Can you work these out from the model? Positions are in its coordinate system, mm. Round coordinates to 2 decimals unless told otherwise and drop trailing zeros. Loops run counter-clockwise (first coordinate to the right, second up) from the corner with the lowest first, then second, coordinate; pieces in that order, holes last.
Autodesk Inventor part; units mm, degrees
ref_plane "YZ Plane" through (0, 0, 0) normal (1, 0, 0) x (0, 1, 0)
ref_plane "XZ Plane" through (0, 0, 0) normal (0, 1, 0) x (-1, 0, 0)
ref_plane "XY Plane" through (0, 0, 0) normal (0, 0, 1) x (1, 0, 0)
sketch "Sketch2" plane through (0, 0, 0) normal (0, 0, 1) x (1, 0, 0)
  line L0 (-7.3607, 82.5814) -> (-7.3607, 22.5627)
  line L1 (-7.3607, 22.5627) -> (0.6393, 28.1644)
  line L2 (0.6393, 28.1644) -> (0.6393, 82.5814)
  line L3 (-7.3607, 82.5814) -> (-10.3607, 82.5814)
  line L4 (-10.3607, 82.5814) -> (-10.3607, 100.5814)
  line L5 (0.6393, 82.5814) -> (3.6393, 82.5814)
  line L6 (3.6393, 82.5814) -> (3.6393, 100.5814)
  line L7 (-10.3607, 100.5814) -> (3.6393, 100.5814)
  line L8 (-10.3607, 85.5814) -> (3.6393, 85.5814) construction
  point P0 (0, 0)
  dimension "d3" = 125
  dimension "d9" = 8
  dimension "d10" = 18
  dimension "d11" = 3
  dimension "d12" = 57.417
  dimension "d13" = 3
  dimension "d14" = 18
extrude "Extrusion1" add sketch "Sketch2" along normal blind 3
sketch "Sketch3" plane through (0, 0, 3) normal (0, 0, 1) x (1, 0, 0)
  line L0 (-10.3607, 100.5814) -> (-10.3607, 82.5814)
  line L1 (3.6393, 82.5814) -> (3.6393, 100.5814)
  line L2 (-10.3607, 85.5814) -> (-7.3607, 85.5814)
  line L3 (-7.3607, 85.5814) -> (-7.3607, 97.5814)
  line L4 (-7.3607, 97.5814) -> (-10.3607, 97.5814)
  line L5 (-10.3607, 97.5814) -> (-10.3607, 85.5814)
  line L6 (3.6393, 85.5814) -> (0.6393, 85.5814)
  line L7 (0.6393, 85.5814) -> (0.6393, 97.5814)
  line L8 (0.6393, 97.5814) -> (3.6393, 97.5814)
  line L9 (3.6393, 97.5814) -> (3.6393, 85.5814)
  point P0 (0, 0)
  dimension "d15" = 3
  dimension "d16" = 12
  dimension "d17" = 3
extrude "Extrusion2" cut sketch "Sketch3" against normal through all
equation "\"d14\" = d10"
properties part number "k2_t_leg"
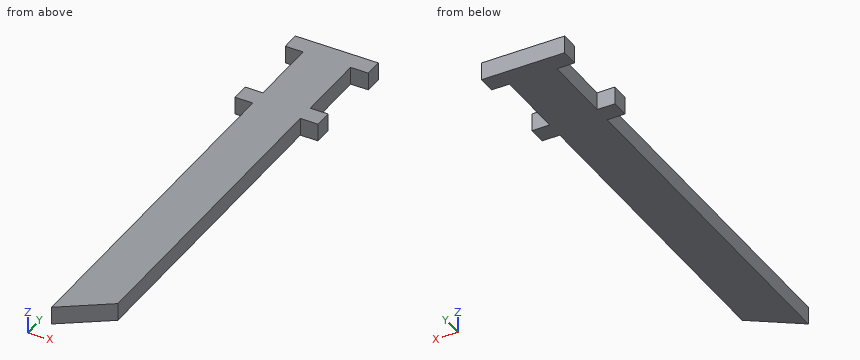
(1) If we section it at B-B, the plane y = 79: List the corners of the cut face in (x, z) for me.
Worked answers:
outline: (-7.36, 0) - (0.64, 0) - (0.64, 3) - (-7.36, 3) - close
(2) If I drill on line 1 (Y direction, x = 1, z = 0.8); line 2 (X direction, y = 29.5, z = 1.35); line 3 (Y direction, x = -0.5, z = 2.45), over which ranges is the centre line in solid material (lowest first)?
Worked answers:
line 1: y = 82.58 to 85.58, 97.58 to 100.58
line 2: x = -7.36 to 0.64
line 3: y = 27.37 to 100.58
(3) Will this pin go through, and if not, where does the flat tip stop? P1, Ø1.5, axis at x = -8.5, z = 1, coming from the -Y side.
Worked answers:
P1: stops at y = 82.58
(4) If we section it at C-C, the plane x = -3: List the corners of the cut face in (y, z) for me.
Worked answers:
outline: (25.62, 0) - (100.58, 0) - (100.58, 3) - (25.62, 3) - close
(5) If we section it at A-A, the plane z = 1.95: List the corners of the cut face in (x, y) for me.
Worked answers:
outline: (-10.36, 82.58) - (-7.36, 82.58) - (-7.36, 22.56) - (0.64, 28.16) - (0.64, 82.58) - (3.64, 82.58) - (3.64, 85.58) - (0.64, 85.58) - (0.64, 97.58) - (3.64, 97.58) - (3.64, 100.58) - (-10.36, 100.58) - (-10.36, 97.58) - (-7.36, 97.58) - (-7.36, 85.58) - (-10.36, 85.58) - close
